Verification items for the finished model (mm, model axes). Round coordinates to 2 decimals unless told otherwise and drop trailing zeros. Write each loop counter-clockwise with the first axis right and the second up, starting at its lowest first coordinate (ties: lowest second). Pieces come first, ordered by that corner, then holes. Notation, with made-up numbers: M 71.5,7.5 L 100.5,7.5 A26 ccw 100.5,22.5 Z; hole C -7.5,41.25 d10. An arc over 180 degrees is marked long. One line per question, with ' | ' between items.
from build123d import *

# Parameters (mm, degrees)
F0_R     = 2.15265
F0_R_2   = 72.39
F0_R_3   = 3.3655
F1_DEPTH = 6.35


with BuildPart() as f1:
    # F0 (on Top) → F1 (new body)
    with BuildSketch(Plane.XY):
        with BuildLine():
            Line((0, 3.175), (0, 0))
            Line((0, 0), (330.2, 0))
            Line((330.2, 0), (330.2, 3.175))
            Line((330.2, 3.175), (242.28583, 135.304837))
            ThreePointArc((242.28583, 135.304837), (165.1, 176.658321), (87.91417, 135.304837))
            Line((87.91417, 135.304837), (0, 3.175))
        make_face()
        with Locations((123.825, 12.457924)):
            Circle(F0_R, mode=Mode.SUBTRACT)
        with Locations((82.55, 83.948321)):
            Circle(F0_R, mode=Mode.SUBTRACT)
        with Locations((206.375, 12.457924)):
            Circle(F0_R, mode=Mode.SUBTRACT)
        with Locations((165.1, 83.948321)):
            Circle(F0_R_2, mode=Mode.SUBTRACT)
        with Locations((247.65, 83.948321)):
            Circle(F0_R, mode=Mode.SUBTRACT)
        with Locations((123.825, 155.438718)):
            Circle(F0_R_3, mode=Mode.SUBTRACT)
        with Locations((206.375, 155.438718)):
            Circle(F0_R_3, mode=Mode.SUBTRACT)
    extrude(amount=F1_DEPTH)


solid = f1.part
1. Mould release check, pull along X, two halves, no side actions. Record for faces 1 (the face through (121.34, 157.71, 3.13)), 2 (the face through (163, 11, 6.35)), 3 (the face through (286.858, 68.315, 3.131)): pulls with the +X half, pulls with the -X half, needs draft (parallel to the pull), parting line crosses it, or undercut.
Results:
face 1: undercut | face 2: needs draft | face 3: pulls with the +X half
2. Section check B-B, the plane y = 147. Record the cut outline in (x, z), then the cut area to 3 significant figures.
Results:
outline: M 97.13,0 L 129.54,0 L 129.54,6.35 L 97.13,6.35 Z; M 200.66,0 L 233.07,0 L 233.07,6.35 L 200.66,6.35 Z | area: 412 mm2
3. Section check A-A, the plane x = 165.1. Record the cut outline in (y, z).
Results:
outline: M 0,0 L 11.56,0 L 11.56,6.35 L 0,6.35 Z; M 156.34,0 L 176.66,0 L 176.66,6.35 L 156.34,6.35 Z
4. Go/stop test with flat-tipped pins: P1, Ø3.5, axis at x = 82.55, y = 83.95, coming from the -Z side; P2, Ø3, axis at x = 79, z = 4.5, coming from the +Y side. Record where each tip stops, or that it passes through.
Results:
P1: passes through | P2: stops at y = 124.16
5. Thickness scan on line 1 (Y direction, x = 82.55, z = 4); line 2 (Y direction, x = 275, z = 2.25); line 3 (X direction, y = 129.5, z = 3). Record the ranges inside material, lowest first.
Results:
line 1: y = 0 to 81.8, 86.1 to 127.24 | line 2: y = 0 to 86.14 | line 3: x = 84.05 to 108.84, 221.36 to 246.15
6. Section check D-D, the plane x = 281. Record the cut outline in (y, z), then the cut area to 3 significant figures.
Results:
outline: M 0,0 L 77.12,0 L 77.12,6.35 L 0,6.35 Z | area: 490 mm2
7. Section check C-C, the plane z = 4. Count the separate pieces of the cut face and the enclosed holes in it, then the cut area to 3 significant figures.
Results:
separate pieces: 1 | enclosed holes: 7 | area: 21,000 mm2
